Verification items for the finished model (mm, model axes). Face numbers are marked on the shaded views. A direction names the side the tool comes from. Give positions to 0.01 mm unless a question says otherwise; leave off trailing zeros. Write each loop counter-clockwise with the first axis right and the second up, starting at its lowest first coordinate (ties: lowest second). Pieces come first, ordered by that corner, then holes. Notation, with made-up numbers: (28, 2.5) -> (77, 2.5) arc R26 cw to (77, 35.5) -> close; hole circle Ø10 at (-5.5, 2.5). An arc over 180 degrees is marked (long way). Use one line per item in the form item = value. Start each with the question number.
(1) Section check A-A, the plane y = 10.5. Record the cut outline in (x, z) (3 decimals).
(2) Section check C-C, the plane x = 9. Record the cut outline in (y, z) (3 decimals).
(3) Scan lines: L1, parallel to Z at x = 16.5, y = -0.5 (3 decimals); L2, parallel to Z at x = 2.5, y = 13 (3 decimals); L3, parallel to X at y = 0.25, z = 10.5. Record each from-to range of solid material in increasing order.
(4) Set-up check for the marked faces 1, 2 and 3: record each of +Z, -Z, +X, -X, +Y, -Y from which the full face is reachable in a straight line by a thin tool's end or side.
(5) Depth check by flat-ended pin: pin 1 Ø5 at (x, z) = (10, -8.5) entering from -Y (3 decimals); pin 2 Ø7.5 at (y, z) = (6.5, -10) entering from +X (3 decimals); pin 3 Ø6.5 at (x, z) = (11.5, 6.5) entering from -Y; pin 4 Ø4 at (x, y) = (9.525, 9.525) entering from -Z. Enter the tip coordinate at first touch or a pass-through.
(6) Section check D-D, the plane z = -5. Record the cut outline in (x, y) (3 decimals).
(7) Section check B-B, the plane x = 14.75. Record the cut outline in (y, z) (3 decimals), plus the area to 3 significant figures.
from build123d import *

# Parameters (mm, degrees)
SKETCH2_W           = 19.05
SKETCH2_H           = 19.05
SKETCH2_R           = 3.175
BOSS_EXTRUDE1_DEPTH = 12.7
SKETCH3_W           = 25.4
SKETCH3_H           = 25.4
BOSS_EXTRUDE2_DEPTH = 3.175
SKETCH4_W           = 12.7
SKETCH4_H           = 12.7
BOSS_EXTRUDE3_DEPTH = 9.525
SKETCH5_R           = 3.175
CUT_EXTRUDE1_DEPTH  = 41.411152545
SKETCH6_R           = 2.413
CUT_EXTRUDE2_DEPTH  = 6.35


with BuildPart() as part:
    # Sketch2 → Boss-Extrude1 (new body)
    with BuildSketch(Plane.XY):
        with Locations((9.525, 9.525)):
            Rectangle(SKETCH2_W, SKETCH2_H)
        with Locations((9.525, 9.525)):
            Circle(SKETCH2_R, mode=Mode.SUBTRACT)
    extrude(amount=BOSS_EXTRUDE1_DEPTH)

    # Sketch3 → Boss-Extrude2 (add)
    with BuildSketch(Plane(origin=(0, 0, 0), x_dir=(-1, 0, 0), z_dir=(0, 0, -1))):
        with Locations((-9.525, 9.525)):
            Rectangle(SKETCH3_W, SKETCH3_H)
    extrude(amount=BOSS_EXTRUDE2_DEPTH)

    # Sketch4 → Boss-Extrude3 (add)
    with BuildSketch(Plane(origin=(0, 0, -3.175), x_dir=(-1, 0, 0), z_dir=(0, 0, -1))):
        with Locations((-9.525, 9.525)):
            Rectangle(SKETCH4_W, SKETCH4_H)
    extrude(amount=BOSS_EXTRUDE3_DEPTH)

    # Sketch5 → Cut-Extrude1 (cut, through all)
    with BuildSketch(Plane.XY.offset(12.7)):
        with Locations((9.525, 9.525)):
            Circle(SKETCH5_R)
    extrude(amount=-CUT_EXTRUDE1_DEPTH, mode=Mode.SUBTRACT)

    # Sketch6 → Cut-Extrude2 (cut)
    with BuildSketch(Plane(origin=(0, 15.875, 0), x_dir=(1, 0, 0), z_dir=(0, 1, 0))):
        with Locations(Location((9.525, 7.9375, 0), (0, 0, 180))):
            Circle(SKETCH6_R)
    extrude(amount=-CUT_EXTRUDE2_DEPTH, mode=Mode.SUBTRACT)


solid = part.part
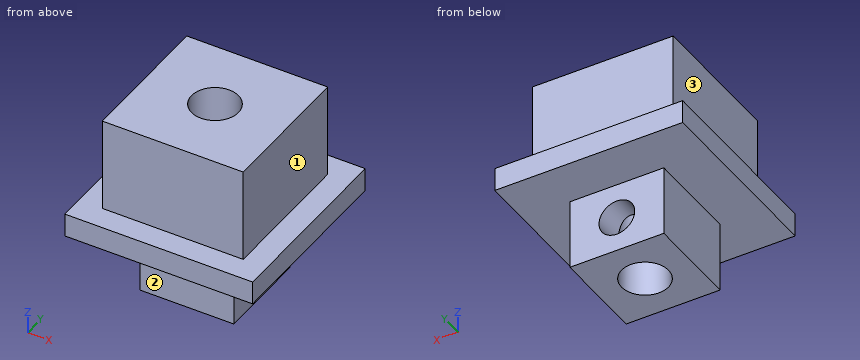
Completed:
q1.outline = (-3.175, -3.175) -> (3.175, -3.175) -> (3.175, -12.7) -> (6.503, -12.7) -> (6.503, 12.7) -> (0, 12.7) -> (0, 0) -> (-3.175, 0) -> close; (12.547, -12.7) -> (15.875, -12.7) -> (15.875, -3.175) -> (22.225, -3.175) -> (22.225, 0) -> (19.05, 0) -> (19.05, 12.7) -> (12.547, 12.7) -> close
q2.outline = (-3.175, -3.175) -> (3.175, -3.175) -> (3.175, -12.7) -> (6.394, -12.7) -> (6.394, 12.7) -> (0, 12.7) -> (0, 0) -> (-3.175, 0) -> close; (12.656, -12.7) -> (15.875, -12.7) -> (15.875, -10.293) -> (12.656, -10.293) -> close; (12.656, -5.582) -> (15.875, -5.582) -> (15.875, -3.175) -> (22.225, -3.175) -> (22.225, 0) -> (19.05, 0) -> (19.05, 12.7) -> (12.656, 12.7) -> close
q3.L1 = -3.175 to 0
q3.L2 = -3.175 to 12.7
q3.L3 = 0 to 19.05
q4.face_1 = +Z, +X, +Y, -Y
q4.face_2 = -Z, +X, -X, -Y
q4.face_3 = +Z, -X, +Y, -Y
q5.pin_1 = 3.175
q5.pin_2 = 15.875
q5.pin_3 = 0
q5.pin_4 = through
q6.outline = (3.175, 3.175) -> (15.875, 3.175) -> (15.875, 15.875) -> (3.175, 15.875) -> close; hole circle Ø6.35 at (9.525, 9.525)
q7.outline = (-3.175, -3.175) -> (3.175, -3.175) -> (3.175, -12.7) -> (15.875, -12.7) -> (15.875, -3.175) -> (22.225, -3.175) -> (22.225, 0) -> (19.05, 0) -> (19.05, 12.7) -> (0, 12.7) -> (0, 0) -> (-3.175, 0) -> close
q7.area = 444 mm²
